Can you work these out from the drawing? Everything is in mm from the part's minimum corner. A direction names the side the tool comes from. Round coordinates to 2 decimals unless told otherwise and drop trailing zeros. Write each loop counter-clockwise with the first axis right and the second up, starting at its lowest first coordinate (ties: lowest second). Pieces come first, ordered by that corner, then holes. Notation, with made-up numbers: (-22, 76.25) - (16, 76.25) arc R32 cw to (16, 114.25) - close; hole circle Ø1 at (7, 79.5). An arc over 180 degrees is marked (long way). Write each question's results on one line, items separated by ' | '. Start each with the question number.
(1) On a 3-axis mill with a long thin cutter (end or side, diameter ignored), from which of +Z, -Z, +X, -X, +Y, -Y can I reach the whole of each face in a straight line? I mean the marked faces 5 and 6. Say none if no direction works.
(2) Imagine slicing it at D-D on x = 25. Write out the boundary of the cut face in (y, z).
(3) Imagine slicing it at B-B on x = 19.5. Write out the boundary of the cut face in (y, z), then the cut area to 3 significant figures.
(4) Imagine slicing it at A-A on z = 11. Write out the boundary of the cut face in (x, y), then the cut area to 3 significant figures.
(5) Please list where these lines run through material, in increasing order: line 1 (Y direction, x = 21.5, z = 28); line 2 (Y direction, x = 25, z = 44); line 3 (X direction, y = 35.5, z = 30.5). Write a range as [from, to].
(6) Thinking about a two-plate mould opening in X: for the marked faces 1, 2, 3 and 4, which applies, +X half, -X half, draft (parallel to the pull), parting line (faces both ways), or undercut?
(7) For P1, Ø6, axis at y = 27.5, z = 62, coming from the +X side; P2, Ø12, axis at x = 7, z = 21, coming from the -Y side; P3, Ø6, axis at y = 37.5, z = 25.5, coming from the +X side; P4, Ø2, axis at x = 38, y = 13.5, coming from the -Z side, each with a flat end and sliding along its axis, tell me the tip position at first contact or that it passes through.
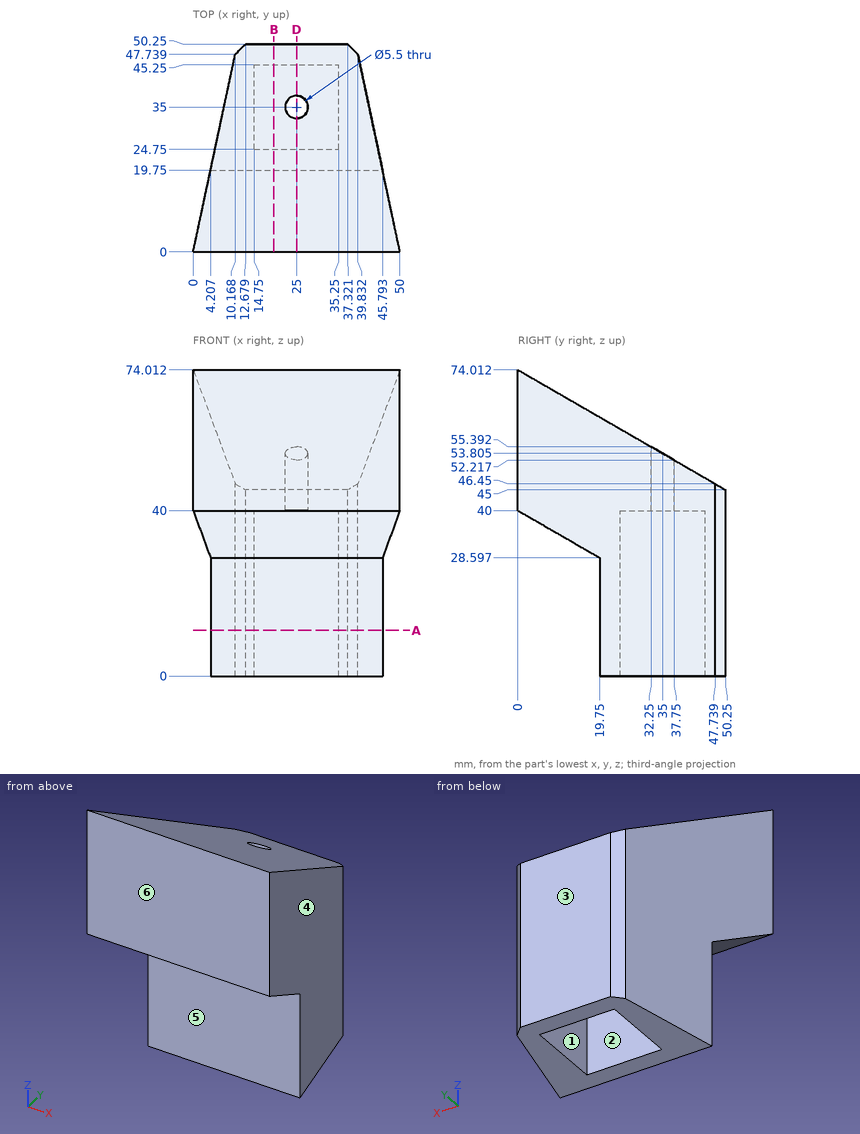
Response:
1) face 5: -Z, +X, -X, -Y | face 6: +Z, -Z, +X, -X, -Y
2) outline: (0, 40) - (19.75, 28.6) - (19.75, 0) - (24.75, 0) - (24.75, 40) - (32.25, 40) - (32.25, 55.39) - (0, 74.01) - close; (37.75, 40) - (45.25, 40) - (45.25, 0) - (50.25, 0) - (50.25, 45) - (37.75, 52.22) - close
3) outline: (0, 40) - (19.75, 28.6) - (19.75, 0) - (24.75, 0) - (24.75, 40) - (45.25, 40) - (45.25, 0) - (50.25, 0) - (50.25, 45) - (0, 74.01) - close | area: 1,490 mm²
4) outline: (4.21, 19.75) - (45.79, 19.75) - (39.83, 47.74) - (37.32, 50.25) - (12.68, 50.25) - (10.17, 47.74) - close; hole (14.75, 24.75) - (35.25, 24.75) - (35.25, 45.25) - (14.75, 45.25) - close | area: 645 mm²
5) line 1: [19.75, 24.75], [45.25, 50.25] | line 2: [0, 32.25], [37.75, 50.25] | line 3: [7.56, 14.75], [35.25, 42.44]
6) face 1: undercut | face 2: undercut | face 3: draft | face 4: +X half
7) P1: through | P2: y = 19.75 | P3: x = 42.65 | P4: z = 31.63
